from build123d import *

# Parameters (mm, degrees)
Y_KSEKLIK_EKSTR_ZYON1_DEPTH = 500
IZIM2_R                     = 4.25
KES_EKSTR_ZYON1_DEPTH       = 10


with BuildPart() as part:
    # Çizim1 → Yükseklik-Ekstrüzyon1 (new body)
    with BuildSketch(Plane.XY):
        Polygon((0, 0), (0, 40), (3, 40), (3, 3), (40, 3), (40, 0), align=None)
    extrude(amount=Y_KSEKLIK_EKSTR_ZYON1_DEPTH)

    # Çizim2 → Kes-Ekstrüzyon1 (cut)
    with BuildSketch(Plane.ZY):
        with Locations((40, 20)):
            Circle(IZIM2_R)
        with Locations((180, 20)):
            Circle(IZIM2_R)
        with Locations((320, 20)):
            Circle(IZIM2_R)
        with Locations((460, 20)):
            Circle(IZIM2_R)
    extrude(amount=-KES_EKSTR_ZYON1_DEPTH, mode=Mode.SUBTRACT)


solid = part.part
The model under review builds one solid part; all positions refer to its coordinate system, in mm. A direction names the side the tool comes from. Give positions to 0.01 mm unless a question says otherwise; leave off trailing zeros. Order: outer loops, then holes, each group sorted by start corner. A loop starts at its lowest first (then second) coordinate and runs counter-clockwise, first axis right, second up. Notation, with made-up numbers: M -39.5,-16.5 L -6.5,-16.5 A22 cw -6.5,1.5 Z; hole C -13.75,41 d5. An arc over 180 degrees is marked long. One line per question, with ' | ' between items. Start each with the question number.
1) Consider section B-B, the plane y = 20. Give the boundary of the cut face in (x, z), then the cut area to 3 significant figures.
2) Clearance check with flat-ended pins moving along their axes: P1, Ø3, axis at y = 13, z = 326, coming from the +X side; P2, Ø10, axis at x = 21.5, z = 59.5, coming from the +Y side. State where each tip first meets the part, or that it passes through.
3) Consider section C-C, the plane x = 31. Give the boundary of the cut face in (y, z).
4) Consider section A-A, the plane z = 180. Give the boundary of the cut face in (x, y), then the cut area to 4 significant figures.
5) For faces 5 (the face through (0, 20, 246)), 6 (the face through (21, 3, 246)), list the 3-axis set-ups (+Z, -Z, +X, -X, +Y, -Y) from which the entire face can be reached by the end or side of a thin tool; tool diameter is ignored.
6) Consider section D-D, the plane z = 280. Give the boundary of the cut face in (x, y), then the cut area to 3 significant figures.
7) Wall thickness on L1, parallel to X at y = 31, z = 221; L2, parallel to Y at x = 1.8, z = 40: over which ranges is each line inside the solid? List them lowest first. Write a range as from..to.
8) Mouldability with a two-part tool opening along Z and no side actions: class faces 1 (the face through (1.48, 17.41, 176.63)), 2 (the face through (11, 2, 0)), 3 (the face through (1.479, 20.187, 35.754)), 4 (the face through (20, 0, 246)) as pulls with the +Z half, pulls with the -Z half, needs draft (parallel to the pull), parting line crosses it, or undercut.
Found:
1) outline: M 0,0 L 3,0 L 3,35.75 L 0,35.75 Z; M 0,44.25 L 3,44.25 L 3,175.75 L 0,175.75 Z; M 0,184.25 L 3,184.25 L 3,315.75 L 0,315.75 Z; M 0,324.25 L 3,324.25 L 3,455.75 L 0,455.75 Z; M 0,464.25 L 3,464.25 L 3,500 L 0,500 Z | area: 1,400 mm²
2) P1: stops at x = 3 | P2: stops at y = 3
3) outline: M 0,0 L 3,0 L 3,500 L 0,500 Z
4) outline: M 0,0 L 40,0 L 40,3 L 3,3 L 3,15.75 L 0,15.75 Z; M 0,24.25 L 3,24.25 L 3,40 L 0,40 Z | area: 205.5 mm²
5) face 5: +Z, -Z, -X, +Y, -Y | face 6: +Z, -Z, +X, +Y
6) outline: M 0,0 L 40,0 L 40,3 L 3,3 L 3,40 L 0,40 Z | area: 231 mm²
7) L1: x = 0..3 | L2: y = 0..15.75, 24.25..40
8) face 1: undercut | face 2: pulls with the -Z half | face 3: undercut | face 4: needs draft
